from build123d import *

# Parameters (mm, degrees)
BOSS_EXTRUDE1_DEPTH = 4.7625
SKETCH2_R           = 7.62
CUT_EXTRUDE1_DEPTH  = 30.099355663


with BuildPart() as part:
    # Sketch1 → Boss-Extrude1 (new, symmetric)
    with BuildSketch(Plane.XY):
        Polygon((0, -6.874076643), (0, 6.874076643), (11.90625, 13.748153285), (23.8125, 6.874076643), (23.8125, -6.874076643), (11.90625, -13.748153285), align=None)
    extrude(amount=BOSS_EXTRUDE1_DEPTH, both=True)

    # Sketch2 → Cut-Extrude1 (cut, through all)
    with BuildSketch(Plane.XY.offset(4.7625)):
        with Locations((11.90625, 0)):
            Circle(SKETCH2_R)
    extrude(amount=-CUT_EXTRUDE1_DEPTH, mode=Mode.SUBTRACT)


solid = part.part
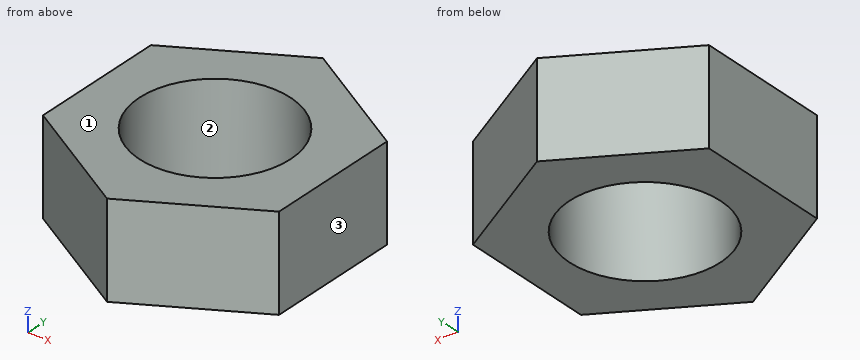
The listing builds one solid part. Answer for the finished solid, in the listing's coordinates (mm). Face numbers are marked on the shaded views. Coordinates: 2 decimals unless noted, no trailing zeros. Loops run counter-clockwise (first coordinate to the right, second up) from the corner with the lowest first, then second, coordinate; pieces in that order, holes last.
1) Find section D-D on y = 8.5. Write down the section's boundary in (x, z), then the cut area to 3 significant figures.
2) Find section B-B on z = 4.25. Write down the section's boundary in (x, y).
3) Find the intervals of material crossed by L1, parallel to X at y = -3.5, z = 1.25; L2, parallel to X at y = 5, z = -3.75; L3, parallel to Y at x = 11, z = 4, in increasing order.
4) Find section C-C on x = 6.25. Write down the section's boundary in (y, z), then the cut area to 3 significant figures.
5) Flat-ended cylindrical pins translate along their axes: pin 1 Ø1.5 at (x, z) = (3, -0.5) entering from -Y; pin 2 Ø12 at (x, y) = (13.5, 5.5) entering from -Z. Find the tip coordinate at first contact, or state that the pin passes through.
6) Find section A-A on y = 0. Write down the section's boundary in (x, z), then the cut area to 3 significant figures.
7) Determine the mould class of the marked faces 1, 2 and 3 for opening direction X: pulls with the +X half, pulls with the -X half, needs draft (parallel to the pull), parting line crosses it, or undercut.
Values:
1. outline: (2.82, -4.76) - (21, -4.76) - (21, 4.76) - (2.82, 4.76) - close
1. area: 173 mm2
2. outline: (0, -6.87) - (11.91, -13.75) - (23.81, -6.87) - (23.81, 6.87) - (11.91, 13.75) - (0, 6.87) - close; hole circle Ø15.24 at (11.91, 0)
3. L1: x = 0 to 5.14, 18.67 to 23.81
3. L2: x = 0 to 6.16, 17.66 to 23.81
3. L3: y = -13.22 to -7.57, 7.57 to 13.22
4. outline: (-10.48, -4.76) - (-5.11, -4.76) - (-5.11, 4.76) - (-10.48, 4.76) - close; (5.11, -4.76) - (10.48, -4.76) - (10.48, 4.76) - (5.11, 4.76) - close
4. area: 102 mm2
5. pin 1: stops at y = -9.04
5. pin 2: stops at z = -4.76
6. outline: (0, -4.76) - (4.29, -4.76) - (4.29, 4.76) - (0, 4.76) - close; (19.53, -4.76) - (23.81, -4.76) - (23.81, 4.76) - (19.53, 4.76) - close
6. area: 81.7 mm2
7. face 1: needs draft
7. face 2: undercut
7. face 3: pulls with the +X half
